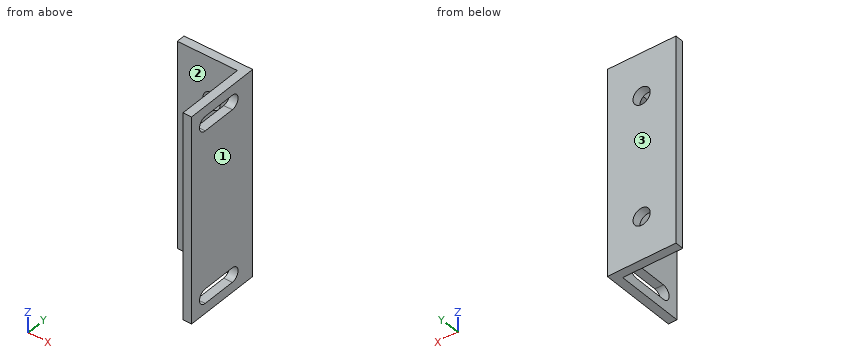
from build123d import *

# Parameters (mm, degrees)
BOSS_EXTRUDE1_DEPTH = 76.2
CUT_EXTRUDE1_REACH  = 97.038
SKETCH2_R           = 3.175
CUT_EXTRUDE2_REACH  = 97.038
SKETCH3_W           = 3.175
SKETCH3_H           = 22.225
CUT_EXTRUDE3_REACH  = 86.362


with BuildPart() as part:
    # Sketch1 → Boss-Extrude1 (new body)
    with BuildSketch(Plane.XY):
        Polygon((0, -50.8), (0, 0), (-25.4, 0), (-25.4, -3.175), (-3.175, -3.175), (-3.175, -50.8), align=None)
    extrude(amount=BOSS_EXTRUDE1_DEPTH)

    # Sketch2 → Cut-Extrude1 (cut, up to next)
    with BuildSketch(Plane(origin=(0, 0, 0), x_dir=(1, 0, 0), z_dir=(0, 1, 0)), mode=Mode.PRIVATE) as cut_extrude1_sk1:
        with Locations(Location((-12.7, -15.875, 0), (0, 0, 270))):
            Circle(SKETCH2_R)
    cut_extrude1_tool1 = extrude(cut_extrude1_sk1.sketch, amount=-CUT_EXTRUDE1_REACH, mode=Mode.PRIVATE) & part.part
    # Sketch2 → Cut-Extrude1 (cut, up to next)
    with BuildSketch(Plane(origin=(0, 0, 0), x_dir=(1, 0, 0), z_dir=(0, 1, 0)), mode=Mode.PRIVATE) as cut_extrude1_sk2:
        with Locations(Location((-12.7, -60.325, 0), (0, 0, 270))):
            Circle(SKETCH2_R)
    cut_extrude1_tool2 = extrude(cut_extrude1_sk2.sketch, amount=-CUT_EXTRUDE1_REACH, mode=Mode.PRIVATE) & part.part
    add(cut_extrude1_tool1.solids().sort_by_distance((-12.7, 0, 15.875))[0], mode=Mode.SUBTRACT)
    add(cut_extrude1_tool2.solids().sort_by_distance((-12.7, 0, 60.325))[0], mode=Mode.SUBTRACT)

    # Sketch3 → Cut-Extrude2 (cut, up to next)
    with BuildSketch(Plane.XY.offset(76.2), mode=Mode.PRIVATE) as cut_extrude2_sk1:
        with Locations((-1.5875, -39.6875)):
            Rectangle(SKETCH3_W, SKETCH3_H)
    cut_extrude2_tool1 = extrude(cut_extrude2_sk1.sketch, amount=-CUT_EXTRUDE2_REACH, mode=Mode.PRIVATE) & part.part
    add(cut_extrude2_tool1.solids().sort_by_distance((-1.5875, -39.6875, 76.2))[0], mode=Mode.SUBTRACT)

    # Sketch4 → Cut-Extrude3 (cut, up to next)
    with BuildSketch(Plane.ZY.offset(3.175), mode=Mode.PRIVATE) as cut_extrude3_sk1:
        with BuildLine():
            Line((72.515, -9.525), (72.515, -22.225))
            ThreePointArc((72.515, -22.225), (69.85, -24.89), (67.185, -22.225))
            Line((67.185, -22.225), (67.185, -9.525))
            ThreePointArc((67.185, -9.525), (69.85, -6.86), (72.515, -9.525))
        make_face()
    cut_extrude3_tool1 = extrude(cut_extrude3_sk1.sketch, amount=-CUT_EXTRUDE3_REACH, mode=Mode.PRIVATE) & part.part
    # Sketch4 → Cut-Extrude3 (cut, up to next)
    with BuildSketch(Plane.ZY.offset(3.175), mode=Mode.PRIVATE) as cut_extrude3_sk2:
        with BuildLine():
            Line((3.685, -9.525), (3.685, -22.225))
            ThreePointArc((3.685, -22.225), (6.35, -24.89), (9.015, -22.225))
            Line((9.015, -22.225), (9.015, -9.525))
            ThreePointArc((9.015, -9.525), (6.35, -6.86), (3.685, -9.525))
        make_face()
    cut_extrude3_tool2 = extrude(cut_extrude3_sk2.sketch, amount=-CUT_EXTRUDE3_REACH, mode=Mode.PRIVATE) & part.part
    add(cut_extrude3_tool1.solids().sort_by_distance((-3.175, -15.875, 69.85))[0], mode=Mode.SUBTRACT)
    add(cut_extrude3_tool2.solids().sort_by_distance((-3.175, -15.875, 6.35))[0], mode=Mode.SUBTRACT)


solid = part.part
For this review, take the finished solid that the model builds, in its own axes (mm). Face numbers are marked on the shaded views. Coordinates: 2 decimals unless noted, no trailing zeros. Order: outer loops, then holes, each group sorted by start corner. A loop starts at its lowest first (then second) coordinate and runs counter-clockwise, first axis right, second up. Notation, with made-up numbers: (51, 46) - (102, 46) arc R18 ccw to (102, 59) - close; hole circle Ø9 at (-19, -26.75). An arc over 180 degrees is marked (long way). Use one line per item in the form item = value.
Q1. Consider section B-B (y = -15.75). Give the boundary of the cut face in (x, z) (3 decimals).
Checked values:
outline = (-3.175, 0) - (0, 0) - (0, 3.685) - (-3.175, 3.685) - close; (-3.175, 9.015) - (0, 9.015) - (0, 67.185) - (-3.175, 67.185) - close; (-3.175, 72.515) - (0, 72.515) - (0, 76.2) - (-3.175, 76.2) - close
Q2. Consider section A-A (x = -12.7). Give the boundary of the cut face in (y, z) (3 decimals).
Checked values:
outline = (-3.175, 0) - (0, 0) - (0, 12.7) - (-3.175, 12.7) - close; (-3.175, 19.05) - (0, 19.05) - (0, 57.15) - (-3.175, 57.15) - close; (-3.175, 63.5) - (0, 63.5) - (0, 76.2) - (-3.175, 76.2) - close
Q3. Consider section C-C (z = 6.35). Give the boundary of the cut face in (x, y) (3 decimals).
Checked values:
outline = (-25.4, -3.175) - (-3.175, -3.175) - (-3.175, -6.86) - (0, -6.86) - (0, 0) - (-25.4, 0) - close; (-3.175, -28.575) - (0, -28.575) - (0, -24.89) - (-3.175, -24.89) - close
Q4. Draft analysis for pull direction Y (two halves, no side actions). For the marked faces 1, 2 and 3, state which applies: +Y half, -Y half, draft (parallel to the pull), parting line (faces both ways), or undercut.
Checked values:
face_1 = draft
face_2 = -Y half
face_3 = +Y half
Q5. For P1, Ø2, axis at y = -7.5, z = 40, coming from the +X side; P2, Ø6.5, axis at x = -14, z = 48.5, coming from the -Y side (3 decimals); P3, Ø4, axis at x = -12.7, z = 15.875, coming from the -Y side; P4, Ø2, axis at y = -20, z = 53.5, coming from the -X side (3 decimals), all flat-tipped, find the tip position at first contact; note any pin that passes through.
Checked values:
P1 = 0
P2 = -3.175
P3 = through
P4 = -3.175
Q6. Consider section D-D (y = -1.75). Give the boundary of the cut face in (x, z) (3 decimals), then the cut area to 3 significant figures.
Checked values:
outline = (-25.4, 0) - (0, 0) - (0, 76.2) - (-25.4, 76.2) - close; hole circle Ø6.35 at (-12.7, 15.875); hole circle Ø6.35 at (-12.7, 60.325)
area = 1,870 mm2
Q7. For probe 1 along Y at (x, z) = (-6, 18.5) (3 decimals); probe 2 along Z at (x, y) = (-1.5, -24.25), list the stretches that pass through material, from the lowest coordinate up. Write a range as from..to.
Checked values:
probe_1 = -3.175..0
probe_2 = 0..4.62, 8.08..68.12, 71.58..76.2
